For this review, take the finished solid that the model builds, in its own axes (mm). Give positions to 0.01 mm unless a question says otherwise; leave off trailing zeros. Write each loop counter-clockwise with the first axis right and the second up, starting at its lowest first coordinate (ties: lowest second). Pieces come first, ordered by that corner, then holes. Notation, with made-up numbers: M 41,8 L 95,8 A12 ccw 95,22 Z; hole C -34,81 d9. An arc over 180 degrees is marked long. Write item = value, one per line.
```python
from build123d import *

# Parameters (mm, degrees)
SKETCH1_R           = 81.2
BOSS_EXTRUDE1_DEPTH = 5
SKETCH4_R           = 14.75
BOSS_EXTRUDE2_DEPTH = 25
CUT_EXTRUDE2_DEPTH  = 118.523955005
CIRPATTERN2_COUNT   = 54
CUT_EXTRUDE4_DEPTH  = 118.337042358
SKETCH5_W           = 5
SKETCH5_H           = 29.5
CUT_EXTRUDE3_DEPTH  = 25
LPATTERN1_COUNT     = 2
LPATTERN1_PITCH     = 90


with BuildPart() as part:
    # Sketch1 → Boss-Extrude1 (new body)
    with BuildSketch(Plane(origin=(0, 0, 0), x_dir=(1, 0, 0), z_dir=(0, 1, 0))):
        with Locations(Location((0, 0, 0), (0, 0, 270))):
            Circle(SKETCH1_R)
    extrude(amount=BOSS_EXTRUDE1_DEPTH)

    # Sketch4 → Boss-Extrude2 (add)
    with BuildSketch(Plane(origin=(0, 5, 0), x_dir=(1, 0, 0), z_dir=(0, 1, 0))):
        with Locations(Location((0, 0, 0), (0, 0, 270))):
            Circle(SKETCH4_R)
    extrude(amount=BOSS_EXTRUDE2_DEPTH)

    # Sketch2 → Cut-Extrude2 (cut, through all)
    with BuildSketch(Plane(origin=(0, 5, 0), x_dir=(1, 0, 0), z_dir=(0, 1, 0))):
        with BuildLine():
            ThreePointArc((5, 81.045912914), (0, 81.2), (-5, 81.045912914))
            ThreePointArc((-5, 81.045912914), (-1.725153292, 79.42244122), (0, 76.2))
            ThreePointArc((0, 76.2), (1.725153292, 79.42244122), (5, 81.045912914))
        make_face()
    cut_extrude2 = extrude(amount=-CUT_EXTRUDE2_DEPTH, mode=Mode.SUBTRACT)

    # CirPattern2: Cut-Extrude2 ×54 about axis
    cirpattern2_axis = Axis((0, 0, 0), (0, 1, 0))
    for i in range(1, CIRPATTERN2_COUNT):
        add(cut_extrude2.rotate(cirpattern2_axis, i * 360 / CIRPATTERN2_COUNT), mode=Mode.SUBTRACT)

    # Sketch6 → Cut-Extrude4 (cut, through all)
    with BuildSketch(Plane(origin=(0, 5, 0), x_dir=(1, 0, 0), z_dir=(0, 1, 0))):
        with BuildLine():
            Line((-58, -2.5), (-32, -2.5))
            ThreePointArc((-32, -2.5), (-30.585786438, -1.914213562), (-30, -0.5))
            Line((-30, -0.5), (-30, 0.5))
            ThreePointArc((-30, 0.5), (-30.585786438, 1.914213562), (-32, 2.5))
            Line((-32, 2.5), (-58, 2.5))
            ThreePointArc((-58, 2.5), (-59.414213562, 1.914213562), (-60, 0.5))
            Line((-60, 0.5), (-60, -0.5))
            ThreePointArc((-60, -0.5), (-59.414213562, -1.914213562), (-58, -2.5))
        make_face()
    cut_extrude4 = extrude(amount=-CUT_EXTRUDE4_DEPTH, mode=Mode.SUBTRACT)

    # Sketch5 → Cut-Extrude3 (cut)
    with BuildSketch(Plane(origin=(0, 30, 0), x_dir=(1, 0, 0), z_dir=(0, 1, 0))):
        Rectangle(SKETCH5_W, SKETCH5_H)
    extrude(amount=-CUT_EXTRUDE3_DEPTH, mode=Mode.SUBTRACT)

    # LPattern1: Cut-Extrude4 ×2
    with Locations(*[(i * LPATTERN1_PITCH, 0, 0) for i in range(1, LPATTERN1_COUNT)]):
        add(cut_extrude4, mode=Mode.SUBTRACT)


solid = part.part
```
1. The part is to be moulded in two halves that separate along Z. For faces 1 (the face through (14.747, 17.325, 0.289)), 2 (the face through (-34.164, 2.535, -71.565)), say which applies: +Z half, -Z half, draft (parallel to the pull), parting line (faces both ways), or undercut.
Responses:
face_1 = parting line
face_2 = undercut
2. We need section A-A, the plane x = 45. Write out the cut boundary in (y, z).
Responses:
outline = M 0,-65.39 L 5,-65.39 L 5,-2.5 L 0,-2.5 Z; M 0,2.5 L 5,2.5 L 5,65.39 L 0,65.39 Z
3. Insertion check: P1, Ø1.5, axis at x = 49, y = 3.5, coming from the -Z side; P2, Ø1.5, axis at x = -32.5, z = -21.5, coming from the +Y side; P3, Ø6, axis at x = -40.5, z = 8, coming from the -Y side; P4, Ø7.5, axis at y = 22.5, z = 1.5, coming from the +X side. Each pin has a flat end and moves straight along its axis. Give the tip position at first contact, or say it passes through.
Responses:
P1 = -65.16
P2 = 5
P3 = 0
P4 = 14.75
4. We need section D-D, the plane x = -20. Write out the cut boundary in (y, z), then the cut area to 3 significant figures.
Responses:
outline = M 0,-76.89 L 5,-76.89 L 5,76.89 L 0,76.89 Z
area = 769 mm2
5. We need section C-C, the plane z = -55.5. Write out the cut boundary in (x, y).
Responses:
outline = M -56.58,0 L 56.58,0 L 56.58,5 L -56.58,5 Z
6. For line 1 along Y through (x, z) = (-54.5, 52.5); line 2 along X through (y, z) = (22.75, -6.5); line 3 along X through (y, z) = (6, -3.5), list the stretches that pass through material, from the lowest coordinate up. Write a range as from..to.
Responses:
line_1 = 0..5
line_2 = -13.24..-2.5, 2.5..13.24
line_3 = -14.33..-2.5, 2.5..14.33
7. We need section B-B, the plane y = 27. Write out the cut boundary in (x, z), then the cut area to 3 significant figures.
Responses:
outline = M -2.5,-14.54 L -2.5,14.54 A14.75 ccw Z; M 2.5,-14.54 A14.75 ccw 2.5,14.54 Z
area = 537 mm2
